CAD build for the part. Positions are in the model's coordinates, mm. Face numbers are marked on the shaded views. Coordinates: 2 decimals unless noted, no trailing zeros. Loops run counter-clockwise (first coordinate to the right, second up) from the corner with the lowest first, then second, coordinate; pieces in that order, holes last. Notation, with made-up numbers: (-31.75, 30) - (-8.75, 30) arc R24 cw to (-8.75, 44) - close; hole circle Ø5 at (-39, 86.25). An arc over 180 degrees is marked (long way). Put each result on its own line as item: value.
```python
from build123d import *

# Parameters (mm, degrees)
FORO_LAMATO_PER_BULLONE_M5_A_TESTA_ESAGO_D           = 5.5
FORO_LAMATO_PER_BULLONE_M5_A_TESTA_ESAGO_DEPTH       = 48
FORO_LAMATO_PER_BULLONE_M5_A_TESTA_ESAGO_CBORE_D     = 12.238
FORO_LAMATO_PER_BULLONE_M5_A_TESTA_ESAGO_CBORE_DEPTH = 3.5
FORO_LAMATO_PER_BULLONE_M5_A_TESTA_ESAGO_TIP         = 1.652366702


with BuildPart() as part:
    # Schizzo1 → Rivoluzione1 (revolve)
    with BuildSketch(Plane.XY):
        Polygon((20, 68), (109, 68), (109, 30), (30, 30), (30, 5), (48, 5), (48, 0), (0, 0), (0, 148), (20, 148), align=None)
    revolve(axis=Axis((0, -1000, 0), (0, 1, 0)))

    # Foro lamato per Bullone M5 a testa esagonale-1
    with Locations(Plane(origin=(0, 0, 0), x_dir=(-1, 0, 0), z_dir=(0, -1, 0))):
        with Locations((0, 38), (-38, 0), (0, -38), (38, 0)):
            CounterBoreHole(FORO_LAMATO_PER_BULLONE_M5_A_TESTA_ESAGO_D / 2, FORO_LAMATO_PER_BULLONE_M5_A_TESTA_ESAGO_CBORE_D / 2, FORO_LAMATO_PER_BULLONE_M5_A_TESTA_ESAGO_CBORE_DEPTH, depth=FORO_LAMATO_PER_BULLONE_M5_A_TESTA_ESAGO_DEPTH)
            with Locations((0, 0, -(FORO_LAMATO_PER_BULLONE_M5_A_TESTA_ESAGO_DEPTH + FORO_LAMATO_PER_BULLONE_M5_A_TESTA_ESAGO_TIP / 2))):  # 118° drill point
                Cone(0, FORO_LAMATO_PER_BULLONE_M5_A_TESTA_ESAGO_D / 2, FORO_LAMATO_PER_BULLONE_M5_A_TESTA_ESAGO_TIP, mode=Mode.SUBTRACT)


solid = part.part
```
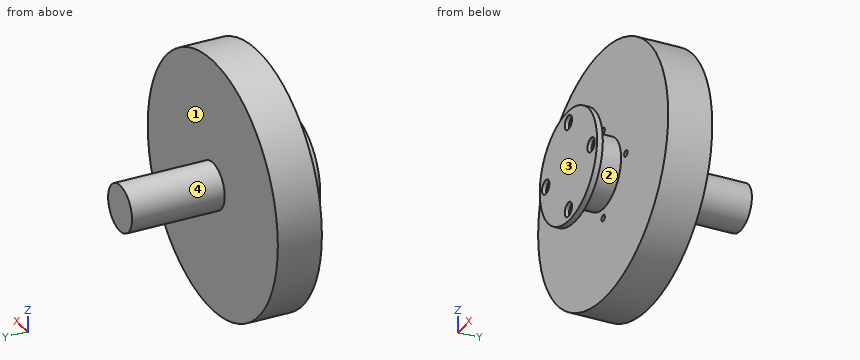
Q1. Mould opens along Y. For the marked faces 1, 2, 3 and 4 say: +Y half, -Y half, draft (parallel to the pull), parting line (faces both ways), or undercut.
Determined:
face 1: +Y half
face 2: undercut
face 3: -Y half
face 4: draft
Q2. Slice it at A-A, the plane y = 41.5. Give the cut face in (x, z), then the cut area to 3 significant figures.
Determined:
outline: circle Ø218 at (0, 0); hole circle Ø5.5 at (-38, 0); hole circle Ø5.5 at (0, -38); hole circle Ø5.5 at (0, 38); hole circle Ø5.5 at (38, 0)
area: 37,200 mm2
Q3. Pin check, flat tips, straight feed: pin 1 Ø10 at (x, z) = (-40, -0.5) entering from -Y; pin 2 Ø5 at (x, y) = (65, 36.5) entering from +Z; pin 3 Ø3.5 at (x, z) = (3, -35.5) entering from -Y; pin 4 Ø19.5 at (x, z) = (-38, 0) entering from +Y. Stop position of each tip, or through.
Determined:
pin 1: y = 0
pin 2: z = 89.3
pin 3: y = 3.5
pin 4: y = 68
Q4. Slice it at B-B, the plane z = 25.5. Give the cut face in (x, y).
Determined:
outline: (-105.98, 30) - (-15.8, 30) - (-15.8, 5) - (-40.67, 5) - (-40.67, 0) - (40.67, 0) - (40.67, 5) - (15.8, 5) - (15.8, 30) - (105.98, 30) - (105.98, 68) - (-105.98, 68) - close
Q5. Slice it at C-C, the plane y = 105. Give the cut face in (x, z), then the cut area to 3 significant figures.
Determined:
outline: circle Ø40 at (0, 0)
area: 1,260 mm2
Q6. Wall check: L1, parallel to Z at x = 0, y = 35; L2, parallel to Z at x = 0, y = 2.35; L3, parallel to Y at x = -58, z = 84. Give the ranges that are in metal, low to high. Write a range as from..to.
Determined:
L1: -109..-40.75, -35.25..35.25, 40.75..109
L2: -48..-44.12, -31.88..31.88, 44.12..48
L3: 30..68
Q7. Slice it at D-D, the plane x = -94. Give the cut face in (y, z).
Determined:
outline: (30, -55.18) - (68, -55.18) - (68, 55.18) - (30, 55.18) - close
